from build123d import *


with BuildPart() as part:
    # 草图1 → 旋转1 (revolve)
    with BuildSketch(Plane.XY, mode=Mode.PRIVATE) as revolve_1_sk:
        with BuildLine():
            Line((0, 0), (0, 1.5))
            Line((0, 1.5), (4, 1.5))
            Line((4, 1.5), (4, 2.3))
            Line((4, 2.3), (6, 2.3))
            Line((6, 2.3), (6, 2.9))
            Line((6, 2.9), (13.1, 2.9))
            ThreePointArc((13.1, 2.9), (13.382842712, 2.782842712), (13.5, 2.5))
            Line((13.5, 2.5), (15.5, 2.5))
            ThreePointArc((15.5, 2.5), (16.207106781, 2.207106781), (16.5, 1.5))
            Line((16.5, 1.5), (16.5, 0))
            Line((16.5, 0), (0, 0))
        make_face()
    revolve(revolve_1_sk.sketch.rotate(Axis((-9.404400031, 0, 0), (1, 0, 0)), 90), axis=Axis((-9.404400031, 0, 0), (1, 0, 0)))


solid = part.part
Input: part model. Units: mm. Frame: model coordinates. A direction names the side the tool comes from. Coordinates: 2 decimals unless noted, no trailing zeros. Loops run counter-clockwise (first coordinate to the right, second up) from the corner with the lowest first, then second, coordinate; pieces in that order, holes last. Notation, with made-up numbers: (59, -16.5) -> (84, -16.5) arc R21 cw to (84, 13.5) -> close; hole circle Ø9 at (67.25, 50.5). An arc over 180 degrees is marked (long way). Write each question's results on one line, items separated by ' | '. Start each with the question number.
Q1. Ray query, line 1 (Y direction, x = 10.75, z = 0.15); line 2 (X direction, y = 0.25, z = -2.1); line 3 (X direction, y = 0.6, z = -1.85). Return the intervals inside material, ascending. Write a range as from..to.
Q2. Pin query (flat end, axial travel): pin 1 (2 mm diameter, centred on x = 13, y = -2, fed in from -Z); pin 2 (1 mm diameter, centred on y = 0, z = -1, fed in from -X). Return the tip coordinate at first contact, or that it passes through.
Q3. Section D-D, the plane x = 11.5. Return the cut outline in (y, z).
Q4. Section A-A, the plane z = 0. Return the cut outline in (x, y), plus the area to 3 significant figures.
Q5. Reachability of faces 1 (the cylindrical face through (9.6, -0.1, -2.9)), 2 (the cylindrical face through (2.03, -0.45, 1.43)), 3 (the cylindrical face through (14.5, -0.1, -2.5)) from +Z, -Z, +X, -X, +Y, -Y: full face, straight path, thin tool, end or side. Return the list, or none.
Q6. Section C-C, the plane x = 5. Return the cut outline in (y, z), plus the area to 3 significant figures.
Found:
1) line 1: -2.9..2.9 | line 2: 4..16.29 | line 3: 4..16.4
2) pin 1: z = -2.72 | pin 2: x = 0
3) outline: circle Ø5.8 at (0, 0)
4) outline: (0, -1.5) -> (4, -1.5) -> (4, -2.3) -> (6, -2.3) -> (6, -2.9) -> (13.1, -2.9) arc R0.4 ccw to (13.5, -2.5) -> (15.5, -2.5) arc R1 ccw to (16.5, -1.5) -> (16.5, 1.5) arc R1 ccw to (15.5, 2.5) -> (13.5, 2.5) arc R0.4 ccw to (13.1, 2.9) -> (6, 2.9) -> (6, 2.3) -> (4, 2.3) -> (4, 1.5) -> (0, 1.5) -> close | area: 79.2 mm2
5) face 1: +X, -X | face 2: -X | face 3: +X
6) outline: circle Ø4.6 at (0, 0) | area: 16.6 mm2
